Can you work these out from the model? Positions are in its coordinate system, mm. Coordinates: 2 decimals unless noted, no trailing zeros. Order: outer loops, then holes, each group sorted by start corner. A loop starts at its lowest first (then second) coordinate and runs counter-clockwise, first axis right, second up. Notation, with made-up numbers: M 77.5,-14.75 L 97.5,-14.75 A31 ccw 97.5,21.25 Z; hole C 30,40 d11. An arc over 180 degrees is marked long. Answer as CSV lines item,"result". Start each with the question number.
1. I need wall thicknesses on line 1 along Y through (x, z) = (2.55, 0.25); line 2 along Y through (x, z) = (4.05, 6); line 3 along X through (y, z) = (0.9, 6.75). Which ranges of each line are inside material? Lowest first, please. Write a range as from..to.
2. If we section it at C-C (x = 2.5): List the corners of the cut face in (y, z) for me (3 decimals).
3. If we section it at B-B (z = -0.75): List the corners of the cut face in (x, y) for me.
4. If we section it at A-A (y = 0.85): List the corners of the cut face in (x, z) for me.
Solid Edge part; units mm, degrees
sketch "Sketch1" plane through (0, 0, 0) normal (0, -1, 0) x (1, 0, 0)
  line L0 (0, 0) -> (0, 6)
  arc A0 (0, 6) -> (5, 6) centre (2.5, 6) cw
  line L1 (5, 6) -> (5, 0)
  arc A1 (0, 0) -> (5, 0) centre (2.5, 0) ccw
extrude "Protrusion1" add sketch "Sketch1" against normal blind 2
sketch "Sketch2" plane through (5, 1, 3) normal (1, 0, 0) x (0, 1, 0)
  line L0 (1, 5.5) -> (0.25, 5.5)
  arc A0 (0.25, 5.5) -> (0.25, -5.5) centre (11.725, 0) ccw
  line L1 (1, -5.5) -> (0.25, -5.5)
  line L2 (1, 5.5) -> (1, -5.5)
extrude "ExtrudedCutout_1" cut sketch "Sketch2" against normal blind 43.2268 flip side to cut
sketch "Sketch3" plane through (2.5, 0, 3) normal (0, -1, 0) x (0, 0, 1)
  arc A0 (-3, 2) -> (-3, -2) centre (-3, 0) ccw
  line L0 (-3, -2) -> (3, -2)
  arc A1 (3, 2) -> (3, -2) centre (3, 0) cw
  line L1 (-3, 2) -> (3, 2)
extrude "ExtrudedCutout_2" cut sketch "Sketch3" against normal blind 3.7815 flip side to cut
sketch "Sketch4" plane through (4.5, 1, 3) normal (1, 0, 0) x (0, 0, 1)
  line L0 (-5, -1) -> (-5, -0.25)
  line L1 (-5, -0.25) -> (5, -0.25)
  line L2 (5, -0.25) -> (5, -1)
  line L3 (5, -1) -> (-5, -1)
extrude "ExtrudedCutout_3" cut sketch "Sketch4" against normal blind 4.4511
properties material "Glass, general industrial"
Solved:
1,line 1,"0.3..1.25"
1,line 2,"0.36..1.25"
1,line 3,"0.65..4.35"
2,outline,"M 1.023,-2 L 1.25,-2 L 1.25,8 L 1.023,8 A12.725 ccw Z"
3,outline,"M 0.65,0.57 L 4.35,0.57 L 4.35,1.25 L 0.65,1.25 Z"
4,outline,"M 0.5,0 A2 ccw 1.26,-1.57 L 3.74,-1.57 A2 ccw 4.5,0 L 4.5,6 A2 ccw 3.74,7.57 L 1.26,7.57 A2 ccw 0.5,6 Z"
